```python
from build123d import *
from build123d.topology import SkipClean

# Parameters (mm, degrees)
SKETCH1_R           = 9
BOSS_EXTRUDE1_DEPTH = 5
SKETCH2_R           = 13.469028944
BOSS_EXTRUDE2_DEPTH = 3
SHELL1_T            = -2
FILLET1_R           = 2
CUT_EXTRUDE1_START  = -13
CUT_EXTRUDE1_DEPTH  = 13


with BuildPart() as part:
    # Sketch1 → Boss-Extrude1 (new body)
    with BuildSketch(Plane(origin=(0, 0, 0), x_dir=(1, 0, 0), z_dir=(0, 1, 0))):
        with Locations(Location((0, 0, 0), (0, 0, 270))):
            Circle(SKETCH1_R)
    extrude(amount=BOSS_EXTRUDE1_DEPTH)

    # Sketch2 → Boss-Extrude2 (add)
    with BuildSketch(Plane.XZ):
        with Locations(Location((0, 0, 0), (0, 0, 270))):
            Circle(SKETCH2_R)
    extrude(amount=BOSS_EXTRUDE2_DEPTH)

    # Shell1
    shell1_openings = [part.faces().sort_by_distance(p)[0] for p in [
        (0, -3, 0),
    ]]
    offset(amount=SHELL1_T, openings=shell1_openings, kind=Kind.INTERSECTION)

    # Fillet1
    fillet1_edges = [part.edges().sort_by_distance(p)[0] for p in [
        (0, 5, -9),
    ]]
    fillet(fillet1_edges, radius=FILLET1_R)

    # Sketch3 → Cut-Extrude1 (cut)
    with SkipClean():  # the faces are left unmerged after this step: merging them gives an invalid solid
        with BuildSketch(Plane(origin=(0, 5, 0), x_dir=(1, 0, 0), z_dir=(0, 1, 0)).offset(CUT_EXTRUDE1_START)):
            with BuildLine():
                Line((5.227613876, -2.944834998), (6.098882855, -3.435640831))
                ThreePointArc((6.098882855, -3.435640831), (0, -7), (-6.098882855, -3.435640831))
                Line((-6.098882855, -3.435640831), (-5.227613876, -2.944834998))
                ThreePointArc((-5.227613876, -2.944834998), (0, -6), (5.227613876, -2.944834998))
            make_face()
            with BuildLine():
                Line((5.227613876, 2.944834998), (6.098882855, 3.435640831))
                ThreePointArc((6.098882855, 3.435640831), (0, 7), (-6.098882855, 3.435640831))
                Line((-6.098882855, 3.435640831), (-5.227613876, 2.944834998))
                ThreePointArc((-5.227613876, 2.944834998), (0, 6), (5.227613876, 2.944834998))
            make_face()
        extrude(amount=CUT_EXTRUDE1_DEPTH, mode=Mode.SUBTRACT)


solid = part.part
```
The listing builds one solid part. Answer for the finished solid, in the listing's coordinates (mm). A direction names the side the tool comes from. Coordinates: 2 decimals unless noted, no trailing zeros. Order: outer loops, then holes, each group sorted by start corner. A loop starts at its lowest first (then second) coordinate and runs counter-clockwise, first axis right, second up. Notation, with made-up numbers: M -15,-20.75 L 25,-20.75 A17 cw 25,-5.75 Z; hole C -2,-21.75 d10. An arc over 180 degrees is marked long. Answer as a JSON object with one key per item and string values. Group by question number.
1. Straight lines are drawn through the part: line 1 (X direction, y = -2.5, z = 0); line 2 (Z direction, x = 1.5, y = 3.5); line 3 (Z direction, x = 2, y = 4.75). For each, find the intervals that lie inside material, in ascending order.
2. Section D-D on y = 4.5 is taken. Write down the section's boundary in (x, z).
3. Section A-A on x = 0 is taken. Write down the section's boundary in (y, z), then the cut area to 3 significant figures.
4. Determine the mould class of faces 1 (the cylindrical face through (2.703, 1.479, 8.584)), 2 (the cylindrical face through (0, 4, 6)), 3 (the flat face through (-9, 0, -3)) for opening direction Z: released by +Z, released by -Z, zero draft, split by the parting line, or undercut.
5. Flat-ended cylindrical pins translate along their axes: P1, Ø13, axis at x = 1, z = 0.5, coming from the -Y side; P2, Ø1, axis at x = -6, y = 0, coming from the -Z side; P3, Ø4, axis at x = 3, y = 3.5, coming from the -Z side. Find the tip coordinate at first contact, or state that the pin passes through.
6. Section B-B on y = -0.75 is taken. Write down the section's boundary in (x, z), then the cut area to 3 significant figures.
7. A tool of negligible diameter and unlimited length cuts with its end or side. For faces 4 (the flat face through (0, 3, 0)), 5 (the cylindrical face through (0, 4, -6)), 6 (the flat face through (0, 5, 0)), from which of +Z, -Z, +X, -X, +Y, -Y can it reach the whole face along a straight path? Write none if from no direction.
8. Section C-C on z = 0 is taken. Write down the section's boundary in (x, y), then the cut area to 3 significant figures.
Values follow:
{
 "1": {"line 1": "-13.47 to -11.47, 11.47 to 13.47", "line 2": "-8.81 to -6.84, -5.81 to 5.81, 6.84 to 8.81", "line 3": "-7.71 to -6.71, -5.66 to 5.66, 6.71 to 7.71"},
 "2": {"outline": "C 0,0 d16.65; hole M -6.1,-3.44 A7 ccw 6.1,-3.44 L 5.23,-2.94 A6 cw -5.23,-2.94 Z; hole M -6.1,3.44 L -5.23,2.94 A6 cw 5.23,2.94 L 6.1,3.44 A7 ccw Z"},
 "3": {"outline": "M -3,-13.47 L 0,-13.47 L 0,-9 L 3,-9 A2 ccw 5,-7 L -2,-7 L -2,-11.47 L -3,-11.47 Z; M -3,11.47 L -2,11.47 L -2,7 L 5,7 A2 ccw 3,9 L 0,9 L 0,13.47 L -3,13.47 Z; M 3,-6 L 5,-6 L 5,6 L 3,6 Z", "area": "72.2 mm2"},
 "4": {"face 1": "split by the parting line", "face 2": "undercut", "face 3": "zero draft"},
 "5": {"P1": "y = -2", "P2": "z = -12.29", "P3": "z = -8.94"},
 "6": {"outline": "C 0,0 d26.94; hole C 0,0 d14", "area": "416 mm2"},
 "7": {"face 4": "-Y", "face 5": "+Y, -Y", "face 6": "+Z, -Z, +X, -X, +Y"},
 "8": {"outline": "M -13.47,-3 L -11.47,-3 L -11.47,-2 L -7,-2 L -7,3 L 7,3 L 7,-2 L 11.47,-2 L 11.47,-3 L 13.47,-3 L 13.47,0 L 9,0 L 9,3 A2 ccw 7,5 L -7,5 A2 ccw -9,3 L -9,0 L -13.47,0 Z", "area": "76.2 mm2"}
}
